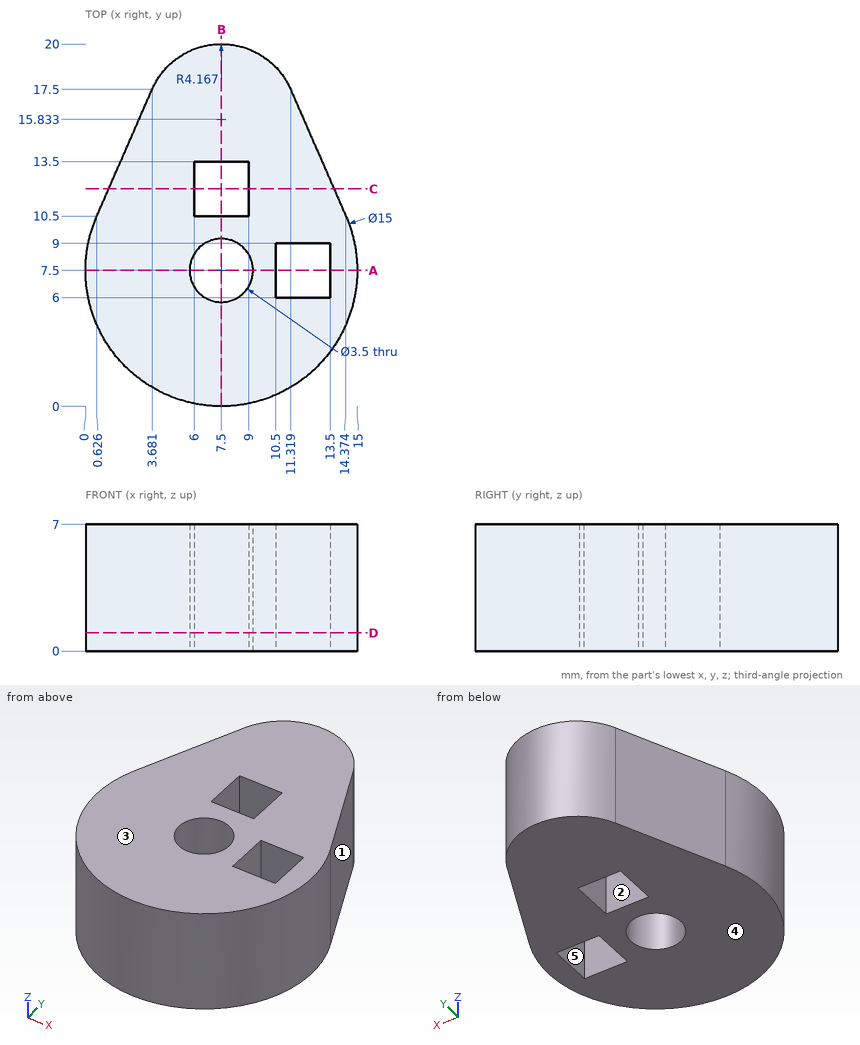
The figure shows three views and two pictorial views of one solid part (mm, origin at its lowest corner). Answer the questions. A direction names the side the tool comes from. Coordinates: 2 decimals unless noted, no trailing zeros. Order: outer loops, then holes, each group sorted by start corner. A loop starts at its lowest first (then second) coordinate and runs counter-clockwise, first axis right, second up. Notation, with made-up numbers: (-12.5, 85.25) - (3.5, 85.25) arc R26 cw to (3.5, 105.25) - close; hole circle Ø5 at (-10, -2.75). An arc over 180 degrees is marked (long way). Answer as a JSON object with one key per item and string values.
1. The mould has two halves that part along X. Classify the marked faces 1, 2 and 3: +X half, -X half, draft (parallel to the pull), parting line (faces both ways), or undercut.
Output values:
{"face 1": "+X half", "face 2": "undercut", "face 3": "draft"}
2. Find section B-B on x = 7.5. Determine the outline of the cut face in (y, z).
Output values:
{"outline": "(0, 0) - (5.75, 0) - (5.75, 7) - (0, 7) - close; (9.25, 0) - (10.5, 0) - (10.5, 7) - (9.25, 7) - close; (13.5, 0) - (20, 0) - (20, 7) - (13.5, 7) - close"}
3. Consider line 1 (Y direction, x = 7.5, z = 1.75); line 2 (X direction, y = 7.75, z = 5.75) (1 decimal); line 3 (Y direction, x = 11, z = 3) (1 decimal). Determine where each line is inside the solid, lowest interval first.
Output values:
{"line 1": "y = 0 to 5.75, 9.25 to 10.5, 13.5 to 20", "line 2": "x = 0 to 5.8, 9.2 to 10.5, 13.5 to 15", "line 3": "y = 0.9 to 6, 9 to 18.1"}
4. Each of these flat-tipped pins is pushed along its axis until it touches: P1, Ø1, axis at y = 4, z = 3.5, coming from the -X side; P2, Ø3.5, axis at y = 12.5, z = 2.5, coming from the -X side (1 decimal); P3, Ø1.5, axis at x = 11.5, z = 4.5, coming from the +Y side. Where does it stop, or does it pass through?
Output values:
{"P1": "stops at x = 0.63", "P2": "stops at x = 0.7", "P3": "stops at y = 18.44"}
5. A tool of negligible diameter and unlimited length cuts with its end or side. For the marked faces 4 and 5, from which of +Z, -Z, +X, -X, +Y, -Y can it reach the whole face along a straight path? Write none if from no direction.
Output values:
{"face 4": "-Z, +X, -X, +Y, -Y", "face 5": "+Z, -Z"}
6. Find section A-A on y = 7.5. Determine the outline of the cut face in (x, z), plus the area to 3 significant figures.
Output values:
{"outline": "(0, 0) - (5.75, 0) - (5.75, 7) - (0, 7) - close; (9.25, 0) - (10.5, 0) - (10.5, 7) - (9.25, 7) - close; (13.5, 0) - (15, 0) - (15, 7) - (13.5, 7) - close", "area": "59.5 mm²"}
7. Find section C-C on y = 12. Determine the outline of the cut face in (x, z).
Output values:
{"outline": "(1.28, 0) - (6, 0) - (6, 7) - (1.28, 7) - close; (9, 0) - (13.72, 0) - (13.72, 7) - (9, 7) - close"}
8. Find section D-D on z = 1. Determine the outline of the cut face in (x, y), plus the area to 3 significant figures.
Output values:
{"outline": "(0.63, 10.5) arc R7.5 ccw (long way) to (14.37, 10.5) - (11.32, 17.5) arc R4.17 ccw to (3.68, 17.5) - close; hole circle Ø3.5 at (7.5, 7.5); hole (6, 10.5) - (9, 10.5) - (9, 13.5) - (6, 13.5) - close; hole (10.5, 6) - (13.5, 6) - (13.5, 9) - (10.5, 9) - close", "area": "193 mm²"}
